```python
from build123d import *

# Parameters (mm, degrees)
F3_DEPTH = 5
F2_W     = 1.972348
F2_H     = 1.531718
F2_W_2   = 0.824641
F2_H_2   = 1.804244
F4_DEPTH = 7
F5_DEPTH = 6
F6_R     = 2.66535
F7_DEPTH = 25


with BuildPart() as f3:
    # F0 (on Top) → F3 (new body)
    with BuildSketch(Plane.XY):
        with BuildLine():
            ThreePointArc((-56.252591, 67.774169), (-58.569985, 66.714597), (-59.516679, 64.348847))
            Line((-59.516679, 64.348847), (-59.516679, 10.507591))
            ThreePointArc((-59.516679, 10.507591), (-58.576435, 8.605541), (-56.804508, 7.438438))
            Line((-56.804508, 7.438438), (-17.379601, 7.438438))
            ThreePointArc((-17.379601, 7.438438), (-15.063115, 8.349842), (-13.988701, 10.59537))
            Line((-13.988701, 10.59537), (-13.988701, 64.895824))
            ThreePointArc((-13.988701, 64.895824), (-15.211268, 66.892462), (-17.3801, 67.774169))
            Line((-17.3801, 67.774169), (-56.252591, 67.774169))
        make_face()
    extrude(amount=F3_DEPTH)

    # F2 (on face) → F4 (join)
    with BuildSketch(Plane.XY):
        Polygon((-34.477703, 47.703966), (-36.762577, 54.855321), (-39.136469, 47.703966), (-46.465863, 47.703966), (-40.501457, 43.371614), (-42.78633, 36.309283), (-36.792252, 40.700983), (-30.768499, 36.309283), (-32.964349, 43.371614), (-27.118638, 47.703966), align=None)
        Polygon((-52.602682, 19.098559), (-54.448072, 19.098559), (-54.448072, 12.837417), (-53.211175, 11.707636), (-51.322754, 11.707636), (-50.25265, 12.837417), (-50.25265, 19.098559), (-51.868297, 19.098559), (-51.868297, 13.260337), (-52.602682, 13.260337), align=None)
        Polygon((-47.797702, 13.197389), (-49.686123, 13.197389), (-49.686123, 11.665671), (-47.776721, 11.665671), align=None)
        with Locations((-41.523952, 12.43153)):
            Rectangle(F2_W, F2_H)
        Polygon((-27.69652, 19.156404), (-29.773781, 19.11444), (-29.773781, 11.665671), (-28.05322, 11.665671), (-28.05322, 16.260827), (-27.297853, 11.665671), (-26.605431, 11.665671), (-25.89203, 16.344756), (-25.89203, 11.665671), (-24.192452, 11.665671), (-24.192452, 19.156404), (-26.33266, 19.156404), (-26.836239, 15.631353), align=None)
        Polygon((-21.800453, 19.156404), (-23.625925, 19.156404), (-22.241084, 15.106793), (-22.241084, 11.707636), (-20.310698, 11.707636), (-20.310698, 15.16974), (-18.946839, 19.11444), (-20.688383, 19.11444), (-21.216365, 16.763071), align=None)
        Polygon((-44.189095, 19.199306), (-46.056628, 19.199306), (-47.21006, 18.192066), (-47.21006, 15.778592), (-46.140123, 14.812943), (-44.838972, 14.812943), (-44.838972, 13.301941), (-45.321684, 13.301941), (-45.321684, 14.162599), (-47.21006, 14.162599), (-47.21006, 12.837417), (-45.92995, 11.707636), (-44.04144, 11.707636), (-42.950634, 12.837417), (-42.950634, 15.00163), (-44.146817, 16.282091), (-45.510922, 16.282091), (-45.510922, 17.814049), (-44.734415, 17.814049), (-44.734415, 16.743535), (-42.929973, 16.743535), (-42.929973, 18.128658), align=None)
        Polygon((-36.5301, 19.199306), (-38.943209, 19.199306), (-39.949652, 11.707636), (-38.250133, 11.707636), (-38.250133, 13.09123), (-37.053928, 13.09123), (-37.053928, 11.707636), (-35.207368, 11.707636), align=None)
        Polygon((-38.125273, 14.558707), (-37.709754, 17.651711), (-37.212875, 14.558707), align=None, mode=Mode.SUBTRACT)
        Polygon((-31.661924, 19.199306), (-34.725517, 19.199306), (-34.725517, 11.707636), (-32.836229, 11.707636), (-32.836229, 14.685798), (-32.186054, 14.685798), (-32.186054, 11.707636), (-30.48607, 11.707636), (-30.48607, 14.727519), (-31.241864, 15.399171), (-30.553139, 16.174177), (-30.553139, 18.127391), align=None)
        with Locations((-32.530801, 16.951129)):
            Rectangle(F2_W_2, F2_H_2, mode=Mode.SUBTRACT)
    extrude(amount=F4_DEPTH)

    # F1 (on face) → F5 (join)
    with BuildSketch(Plane.XY):
        with BuildLine():
            ThreePointArc((-56.361381, 66.743255), (-57.818165, 66.035044), (-58.408085, 64.526476))
            Line((-58.408085, 64.526476), (-58.408085, 27.996894))
            ThreePointArc((-58.408085, 27.996894), (-57.826971, 26.523854), (-56.396667, 25.844317))
            Line((-56.396667, 25.844317), (-17.262138, 25.844317))
            ThreePointArc((-17.262138, 25.844317), (-15.731986, 26.565248), (-15.109562, 28.138047))
            Line((-15.109562, 28.138047), (-15.109562, 64.555392))
            ThreePointArc((-15.109562, 64.555392), (-15.701004, 66.053371), (-17.156273, 66.743255))
            Line((-17.156273, 66.743255), (-56.361381, 66.743255))
        make_face()
        with BuildLine():
            ThreePointArc((-56.961637, 64.553842), (-56.761735, 65.153459), (-56.183666, 65.409072))
            Line((-56.183666, 65.409072), (-17.366143, 65.409072))
            ThreePointArc((-17.366143, 65.409072), (-16.761555, 65.118493), (-16.610773, 64.464867))
            Line((-16.610773, 64.464867), (-16.610773, 28.233234))
            ThreePointArc((-16.610773, 28.233234), (-16.877061, 27.549546), (-17.535625, 27.226076))
            Line((-17.535625, 27.226076), (-56.227252, 27.226076))
            ThreePointArc((-56.227252, 27.226076), (-56.792806, 27.486884), (-56.961637, 28.086357))
            Line((-56.961637, 28.086357), (-56.961637, 64.553842))
        make_face(mode=Mode.SUBTRACT)
        Polygon((-32.648411, 50.138444), (-36.847699, 62.524572), (-40.870544, 50.279595), (-54.033015, 50.279595), (-43.411288, 42.410344), (-47.504712, 29.847771), (-36.81241, 37.646446), (-26.225971, 29.883061), (-30.142954, 42.410344), (-19.66238, 50.138444), align=None)
        Polygon((-39.882477, 48.762206), (-36.847699, 58.501728), (-33.707052, 48.779701), (-23.472983, 48.779701), (-31.625055, 42.833801), (-28.696308, 33.363523), (-36.847699, 39.341208), (-44.928677, 33.447161), (-41.788034, 42.869091), (-49.727861, 48.762206), align=None, mode=Mode.SUBTRACT)
        with BuildLine():
            Line((-17.296651, 22.409985), (-56.159921, 22.409985))
            ThreePointArc((-56.159921, 22.409985), (-57.73311, 21.827224), (-58.39467, 20.285513))
            Line((-58.39467, 20.285513), (-58.39467, 10.552553))
            ThreePointArc((-58.39467, 10.552553), (-57.814134, 9.136198), (-56.406535, 8.534743))
            Line((-56.406535, 8.534743), (-17.266981, 8.534743))
            ThreePointArc((-17.266981, 8.534743), (-15.755662, 9.136305), (-15.071128, 10.611899))
            Line((-15.071128, 10.611899), (-15.071128, 20.137144))
            ThreePointArc((-15.071128, 20.137144), (-15.706151, 21.741357), (-17.296651, 22.409985))
        make_face()
        with BuildLine():
            Line((-57.029683, 10.789941), (-57.029683, 20.018449))
            ThreePointArc((-57.029683, 20.018449), (-56.638588, 20.841056), (-55.753719, 21.057026))
            Line((-55.753719, 21.057026), (-17.534047, 21.057026))
            ThreePointArc((-17.534047, 21.057026), (-16.703582, 20.68187), (-16.43612, 19.810732))
            Line((-16.43612, 19.810732), (-16.43612, 10.878962))
            ThreePointArc((-16.43612, 10.878962), (-16.733474, 10.175971), (-17.445026, 9.899732))
            Line((-17.445026, 9.899732), (-56.169149, 9.899732))
            ThreePointArc((-56.169149, 9.899732), (-56.788219, 10.162327), (-57.029683, 10.789941))
        make_face(mode=Mode.SUBTRACT)
    extrude(amount=F5_DEPTH)

    # F6 (on face) → F7 (cut)
    with BuildSketch(Plane.XY.offset(5)):
        with Locations((-53.391658, 62.098049)):
            Circle(F6_R)
    extrude(amount=-F7_DEPTH, mode=Mode.SUBTRACT)


solid = f3.part
```
Geometry check sheet. Reference: the model listing, model coordinates, mm. A direction names the side the tool comes from. Give positions to 0.01 mm unless a question says otherwise; leave off trailing zeros. Order: outer loops, then holes, each group sorted by start corner. A loop starts at its lowest first (then second) coordinate and runs counter-clockwise, first axis right, second up. Notation, with made-up numbers: (2, 32) - (7, 32) arc R17 ccw to (7, 37) - close; hole circle Ø3 at (-26.5, 52.5). An arc over 180 degrees is marked (long way). Answer in a Markdown table with one row per item. Add a question column.
Q1. Material ranges on probe 1 along X at (y, z) = (56, 5.75); probe 2 along Z at (x, y) = (-38, 52); probe 3 along X at (y, z) = (48, 5.25), recorded low to high. Write a range as from..to.
Q2. Mould release check, pull along Z, two halves, no side actions. Record for faces 1 (the flat face through (-37, 9, 6)), 2 (the flat face through (-43.6, 18.7, 6)): pulls with the +Z half, pulls with the -Z half, needs draft (parallel to the pull), parting line crosses it, or undercut.
Q3. Gauge pin test, flat ends, axial feed: pin 1 (0.8 mm diameter, centred on y = 16, z = 5.5, fed in from +X); pin 2 (1.5 mm diameter, centred on x = -54, z = 6, fed in from +Y); pin 3 (1.6 mm diameter, centred on y = 14.5, z = 6.5, fed in from -X). Record the tip position at first contact, or that the pin passes through.
Q4. Cross-section at A-A, the plane y = 44.5. Enter the section's corners in (x, z).
Q5. Cross-section at C-C, the plane y = 56. Enter the section's corners in (x, z).
Q6. Tool access check on faces 3 (the cylindrical face through (-58.545, 66.741, 2.465)), 4 (the flat face through (-39.44, 15.51, 5.99)). Record the directions out of +Z, -Z, +X, -X, +Y, -Y that give a thin tool (end or side, any length) a straight path to the whole face; none if there is none.
Check values:
| question | item | result |
|---|---|---|
| 1 | probe 1 | x = -58.41..-56.96, -38.99..-37.63, -36.04..-34.64, -16.61..-15.11 |
| 1 | probe 2 | z = 0..5 |
| 1 | probe 3 | x = -58.41..-56.96, -50.96..-48.7, -39.04..-34.57, -24.54..-22.56, -16.61..-15.11 |
| 2 | face 1 | pulls with the +Z half |
| 2 | face 2 | needs draft |
| 3 | pin 1 | stops at x = -15.07 |
| 3 | pin 2 | stops at y = 66.74 |
| 3 | pin 3 | stops at x = -58.39 |
| 4 | outline | (-59.52, 0) - (-13.99, 0) - (-13.99, 5) - (-15.11, 5) - (-15.11, 6) - (-16.61, 6) - (-16.61, 5) - (-27.31, 5) - (-27.31, 6) - (-29.34, 6) - (-29.34, 5) - (-31.44, 5) - (-31.44, 7) - (-42.05, 7) - (-42.05, 5) - (-43.99, 5) - (-43.99, 6) - (-46.23, 6) - (-46.23, 5) - (-56.96, 5) - (-56.96, 6) - (-58.41, 6) - (-58.41, 5) - (-59.52, 5) - close |
| 5 | outline | (-59.52, 0) - (-13.99, 0) - (-13.99, 5) - (-15.11, 5) - (-15.11, 6) - (-16.61, 6) - (-16.61, 5) - (-34.64, 5) - (-34.64, 6) - (-36.04, 6) - (-36.04, 5) - (-37.63, 5) - (-37.63, 6) - (-38.99, 6) - (-38.99, 5) - (-56.96, 5) - (-56.96, 6) - (-58.41, 6) - (-58.41, 5) - (-59.52, 5) - close |
| 6 | face 3 | +Z, -Z, -X, +Y |
| 6 | face 4 | +Z |
